Autodesk Inventor part; units mm, degrees
ref_plane "Work Plane1" through (0, 9.652, 0) normal (0, 1, 0) x (-1, 0, 0)
ref_plane "YZ Plane" through (0, 0, 0) normal (1, 0, 0) x (0, 1, 0)
ref_plane "XY Plane" through (0, 0, 0) normal (0, 0, 1) x (1, 0, 0)
sketch "Sketch1" plane through (0, 0, 0) normal (0, 1, 0) x (-1, 0, 0)
  circle A0 centre (0, 0) radius 12.7
  circle A1 centre (0, 0) radius 2.2225
  dimension "d0" = 25.4
  dimension "d1" = 4.445
ref_plane "Work Plane1" through (0, 9.652, 0) normal (0, 1, 0) x (-1, 0, 0)
sketch "Sketch2" plane through (0, 9.652, 0) normal (0, 1, 0) x (-1, 0, 0)
  circle A0 centre (0, 0) radius 2.2238
  circle A1 centre (0, 0) radius 10.541
  dimension "d3" = 21.082
loft "Loft1" add profiles "Sketch1", "Sketch2" contours A0 | A1 / A0 | A1
sketch "Sketch3" plane through (0, 9.652, 0) normal (0, 1, 0) x (1, 0, 0)
  circle A0 centre (0, 0) radius 2.2225
  dimension "d8" = 4.445
extrude "Extrusion1" cut sketch "Sketch3" against normal blind 25.4
sketch "Sketch4" plane through (0, 9.652, 0) normal (0, 1, 0) x (1, 0, 0)
  circle A0 centre (0, 0) radius 4.8895
  dimension "d11" = 9.779
extrude "Extrusion2" cut sketch "Sketch4" against normal blind 6.096
fillet "Fillet1" radius 0.762 2 edges at (10.541, 9.652, 0) (-4.8895, 3.556, 0)
properties part number "Soft Feet" material "Polystyrene, High Impact"
Part model, mm, in its own coordinate system. A direction names the side the tool comes from. Give positions to 0.01 mm unless a question says otherwise; leave off trailing zeros. Order: outer loops, then holes, each group sorted by start corner. A loop starts at its lowest first (then second) coordinate and runs counter-clockwise, first axis right, second up. Notation, with made-up numbers: (69, 16.25) - (122, 16.25) arc R35 cw to (122, 53.25) - close; hole circle Ø6 at (-4, 79). An arc over 180 degrees is marked (long way). One line per question, with ' | ' between items.
1. Band-saw the part on A-A on x = 0. List the corners of the cut face in (y, z), then the cut area to 3 significant figures.
Filled in:
outline: (0, -12.7) - (9.06, -10.67) arc R0.76 ccw to (9.65, -9.93) - (9.65, -4.89) - (4.32, -4.89) arc R0.76 cw to (3.56, -4.13) - (3.56, -2.22) - (0, -2.22) - close; (0, 2.22) - (3.56, 2.22) - (3.56, 4.13) arc R0.76 cw to (4.32, 4.89) - (9.65, 4.89) - (9.65, 9.93) arc R0.76 ccw to (9.06, 10.67) - (0, 12.7) - close | area: 149 mm²
2. Band-saw the part on B-B on y = 3. List the corners of the cut face in (x, z) (1 decimal), then the cut area to 3 significant figures.
Filled in:
outline: circle Ø24.1 at (0, 0); hole circle Ø4.4 at (0, 0) | area: 439 mm²
3. Pull direction X, two halves, no side cores. Call faces 1 (the face through (-6.049, 6.477, -9.487)), 2 (the face through (2, 3.556, 2)), 3 (the face through (-3, 0, 0)): +X half, -X half, draft (parallel to the pull), parting line (faces both ways), or undercut.
Filled in:
face 1: parting line | face 2: undercut | face 3: draft
4. Drill centre lines: probe 1 along Z at (x, y) = (-4, 9); probe 2 along Z at (x, y) = (0, 0.85); probe 3 along X at (y, z) = (5.75, -1.5). Where is each one in solid material? Low to high.
Filled in:
probe 1: -9.91 to -2.81, 2.81 to 9.91 | probe 2: -12.51 to -2.22, 2.22 to 12.51 | probe 3: -11.31 to -4.65, 4.65 to 11.31
5. Drop flat-ended pins along their axis: P1, Ø10, axis at x = 2.5, z = -8, coming from the -Y side; P2, Ø2, axis at x = -8.5, y = 8.5, coming from the +Z side; P3, Ø3.5, axis at x = 0, z = 0, coming from the +Y side; P4, Ø2, axis at x = 10, y = 4, coming from the -Z side. Give the stop position or say it passes through.
Filled in:
P1: y = 0 | P2: z = 7.82 | P3: through | P4: z = -7.69
6. Which spindle directions (+Z, -Z, +X, -X, +Y, -Y) get a long thin tool onto all of the face, cutting with end or side? Do faces 4 (the face through (5, 9.652, -2)), 5 (the face through (-1.06, 7.022, 4.773)). Say none if no direction does.
Filled in:
face 4: +Z, -Z, +X, -X, +Y | face 5: +Y
